The figure shows three views and two pictorial views of one solid part (mm, origin at its lowest corner). Answer the questions. A direction names the side the tool comes from. Give positions to 0.01 mm unless a question says otherwise; leave off trailing zeros. Write each loop counter-clockwise with the first axis right and the second up, starting at its lowest first coordinate (ties: lowest second). Pieces come first, ordered by that corner, then holes. Notation, with made-up numbers: (7, -35.5) - (22, -35.5) arc R6 cw to (22, -27.5) - close; hole circle Ø3 at (78, -13). An arc over 180 degrees is marked (long way). Write each question's results on one line, items separated by ' | '. Start each with the question number.
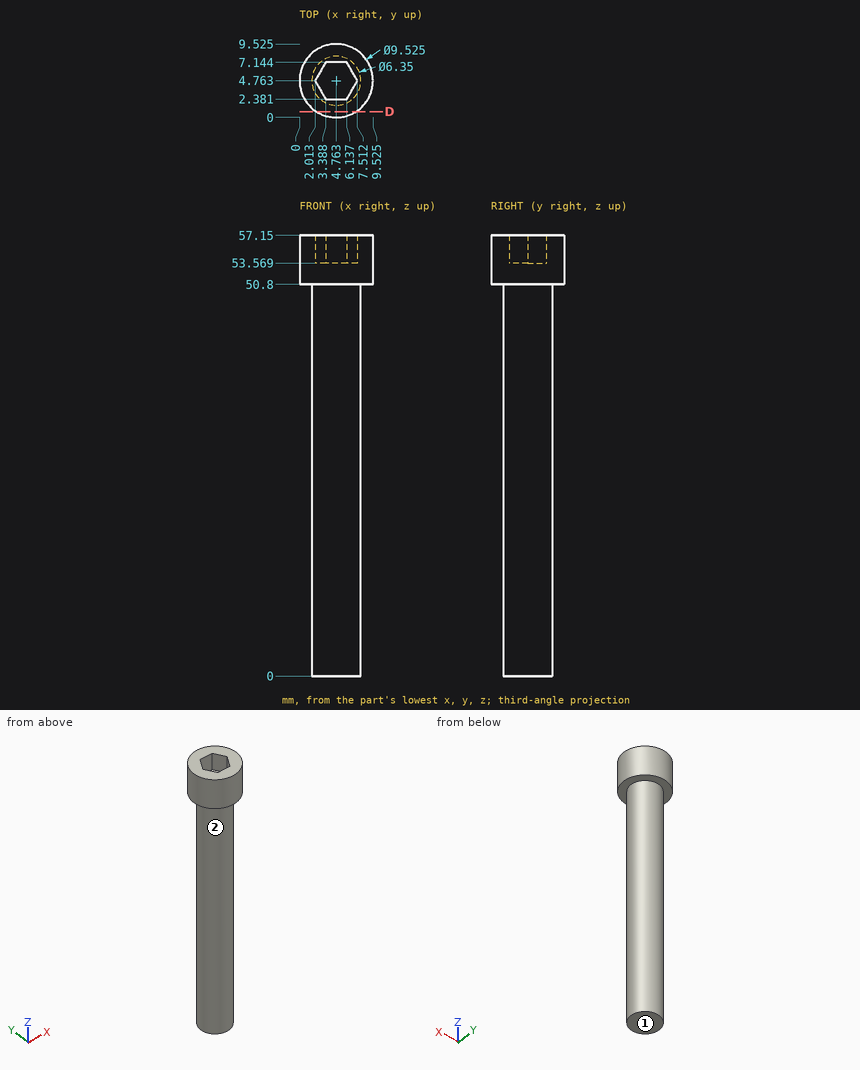
Q1. A cutting plane is placed at D-D, the plane y = 0.75. Write down the section's boundary in (x, z).
Q2. Given pin 1 (4 mm diameter, centred on x = 7.5, z = 9.5, fed in from +Y); pin 2 (3 mm diameter, centred on x = 3.5, z = 33, fed in from -Y); pin 3 (1.5 mm diameter, centred on y = 6.5, z = 18, fed in from -X) (1 decimal), each flat-ended and moving along its own axis, determine where each tip first touches the part or whether it passes through.
Q3. Consider L1, parallel to Z at x = 6.75, y = 3.75; L2, parallel to Z at x = 7.75, y = 7.5; L3, parallel to X at y = 5, z = 8.5. Determine where each line is inside the solid, lowest interval first.
Q4. A tool of negligible diameter and unlimited length cuts with its end or side. For the marked faces 1 and 2, from which of +Z, -Z, +X, -X, +Y, -Y can it reach the whole face along a straight path? Write none if from no direction.
Result:
1) outline: (2.2, 50.8) - (7.33, 50.8) - (7.33, 57.15) - (2.2, 57.15) - close
2) pin 1: stops at y = 7.85 | pin 2: stops at y = 1.59 | pin 3: stops at x = 1.7
3) L1: z = 0 to 53.57 | L2: z = 50.8 to 57.15 | L3: x = 1.6 to 7.93
4) face 1: -Z, +X, -X, +Y, -Y | face 2: -Z
